```python
from build123d import *

# Parameters (mm, degrees)
SKETCH1_R               = 144.4625
BOSS_EXTRUDE1_DEPTH     = 6.35
F_1_4_CLEARANCE_HOLE1_D = 7.14248
SKETCH4_R               = 130.175
SKETCH4_R_2             = 123.825
BOSS_EXTRUDE2_DEPTH     = 63.5
SKETCH7_R               = 120.65
CUT_EXTRUDE1_DEPTH      = 69.85
CUT_EXTRUDE2_REACH      = 220.049
SKETCH8_R               = 38.1


with BuildPart() as part:
    # Sketch1 → Boss-Extrude1 (new body)
    with BuildSketch(Plane(origin=(0, 0, 0), x_dir=(1, 0, 0), z_dir=(0, 1, 0))):
        with Locations(Location((0, 0, 0), (0, 0, 270))):
            Circle(SKETCH1_R)
    boss_extrude1 = extrude(amount=BOSS_EXTRUDE1_DEPTH)

    # 1/4 Clearance Hole1 (through all)
    with Locations(Plane(origin=(0, 6.35, 0), x_dir=(1, 0, 0), z_dir=(0, 1, 0))):
        with Locations((-96.537753301, 96.537753301), (0, 136.525), (96.537753301, 96.537753301), (136.525, 0), (96.537753301, -96.537753301), (0, -136.525), (-96.537753301, -96.537753301), (-136.525, 0)):
            f_1_4_clearance_hole1 = Hole(F_1_4_CLEARANCE_HOLE1_D / 2)

    # Sketch4 → Boss-Extrude2 (add)
    with BuildSketch(Plane(origin=(0, 6.35, 0), x_dir=(1, 0, 0), z_dir=(0, 1, 0))):
        with Locations(Location((0, 0, 0), (0, 0, 270))):
            Circle(SKETCH4_R)
        with Locations(Location((0, 0, 0), (0, 0, 270))):
            Circle(SKETCH4_R_2, mode=Mode.SUBTRACT)
    extrude(amount=BOSS_EXTRUDE2_DEPTH)

    # Mirror2: Boss-Extrude1 across plane
    add(boss_extrude1.mirror(Plane.ZX.offset(38.1)))

    # Mirror3: 1/4 Clearance Hole1 across plane
    add(f_1_4_clearance_hole1.mirror(Plane.ZX.offset(38.1)), mode=Mode.SUBTRACT)

    # Sketch7 → Cut-Extrude1 (cut)
    with BuildSketch(Plane.XZ):
        with Locations(Location((0, 0, 0), (0, 0, 270))):
            Circle(SKETCH7_R)
    extrude(amount=-CUT_EXTRUDE1_DEPTH, mode=Mode.SUBTRACT)

    # Sketch8 → Cut-Extrude2 (cut, up to next)
    with BuildSketch(Plane(origin=(0, 76.2, 0), x_dir=(1, 0, 0), z_dir=(0, 1, 0)), mode=Mode.PRIVATE) as cut_extrude2_sk1:
        with Locations(Location((0, 0, 0), (0, 0, 270))):
            Circle(SKETCH8_R)
    cut_extrude2_tool1 = extrude(cut_extrude2_sk1.sketch, amount=-CUT_EXTRUDE2_REACH, mode=Mode.PRIVATE) & part.part
    add(cut_extrude2_tool1.solids().sort_by_distance((0, 76.2, 0))[0], mode=Mode.SUBTRACT)


solid = part.part
```
Build history of the part. All positions in model axes, mm. A direction names the side the tool comes from. Coordinates: 2 decimals unless noted, no trailing zeros. Order: outer loops, then holes, each group sorted by start corner. A loop starts at its lowest first (then second) coordinate and runs counter-clockwise, first axis right, second up. Notation, with made-up numbers: (40, 51) -> (80, 51) arc R9 cw to (80, 56) -> close; hole circle Ø6 at (76.25, 38). An arc over 180 degrees is marked (long way). Answer in a Markdown table with one row per item. Add a question column.
Q1. Band-saw the part on D-D, the plane y = 17. List the corners of the cut face in (x, z) (3 decimals).
Q2. Band-saw the part on B-B, the plane z = 0. Give the number of separate pieces and of enclosed holes in the cut face, then the cut area to 3 significant figures.
Q3. Drop flat-ended pins along their axis: pin 1 (5.5 mm diameter, centred on x = -96.54, z = 96.54, fed in from -Y); pin 2 (6 mm diameter, centred on x = -48.5, z = -34, fed in from -Y); pin 3 (1.5 mm diameter, centred on y = 52, z = 92, fed in from -X); pin 4 (2 mm diameter, centred on y = 66.5, z = 45.5, fed in from +X). Give the stop position or say it passes through.
Q4. Wall check: line 1 along Y through (x, z) = (-121, 10); line 2 along Z through (x, y) = (-38.5, 27); line 3 along X through (y, z) = (65.5, 9). Give the ranges that are in metal, low to high. Write a range as [from, to].
Q5. Band-saw the part on A-A, the plane x = 7.5. List the corners of the cut face in (y, z).
Q6. Mould opens along X. For faces 1 (the face through (-133.89, 73.07, -2.41)), 2 (the face through (43.393, 3.131, 137.791)), 3 (the face through (-98.46, 73.07, 93.53)), 4 (the face through (108, 6.35, -76)) say: +X half, -X half, draft (parallel to the pull), parting line (faces both ways), or undercut.
Q7. Which spindle directions (+Z, -Z, +X, -X, +Y, -Y) get a long thin tool onto all of the face, cutting with end or side? Do faces 5 (the face through (0.774, 73.069, -133.039)), 6 (the face through (5.305, 3.131, 120.533)), 7 (the face through (129.067, 37.656, -16.946)). Say none if no direction does.
Q8. Band-saw the part on C-C, the plane x = 52. List the corners of the cut face in (y, z), then the cut area to 3 significant figures.
Answers follow:
| question | item | result |
|---|---|---|
| 1 | outline | circle Ø260.35 at (0, 0); hole circle Ø247.65 at (0, 0) |
| 2 | separate pieces | 6 |
| 2 | enclosed holes | 0 |
| 2 | area | 2,280 mm^2 |
| 3 | pin 1 | through |
| 3 | pin 2 | y = 69.85 |
| 3 | pin 3 | x = -92.84 |
| 3 | pin 4 | x = 122.33 |
| 4 | line 1 | [0, 6.35], [69.85, 76.2] |
| 4 | line 2 | [-124.35, -117.69], [117.69, 124.35] |
| 4 | line 3 | [-129.86, -123.5], [123.5, 129.86] |
| 5 | outline | (0, -144.27) -> (6.35, -144.27) -> (6.35, -129.96) -> (69.85, -129.96) -> (69.85, -144.27) -> (76.2, -144.27) -> (76.2, -37.35) -> (69.85, -37.35) -> (69.85, -123.6) -> (6.35, -123.6) -> (6.35, -120.42) -> (0, -120.42) -> close; (0, 120.42) -> (6.35, 120.42) -> (6.35, 123.6) -> (69.85, 123.6) -> (69.85, 37.35) -> (76.2, 37.35) -> (76.2, 144.27) -> (69.85, 144.27) -> (69.85, 129.96) -> (6.35, 129.96) -> (6.35, 144.27) -> (0, 144.27) -> close |
| 6 | face 1 | undercut |
| 6 | face 2 | parting line |
| 6 | face 3 | undercut |
| 6 | face 4 | draft |
| 7 | face 5 | +Y, -Y |
| 7 | face 6 | -Y |
| 7 | face 7 | none |
| 8 | outline | (0, -134.78) -> (6.35, -134.78) -> (6.35, -119.34) -> (69.85, -119.34) -> (69.85, -134.78) -> (76.2, -134.78) -> (76.2, 134.78) -> (69.85, 134.78) -> (69.85, 119.34) -> (6.35, 119.34) -> (6.35, 134.78) -> (0, 134.78) -> (0, 108.87) -> (6.35, 108.87) -> (6.35, 112.38) -> (69.85, 112.38) -> (69.85, -112.38) -> (6.35, -112.38) -> (6.35, -108.87) -> (0, -108.87) -> close |
| 8 | area | 2,920 mm^2 |
